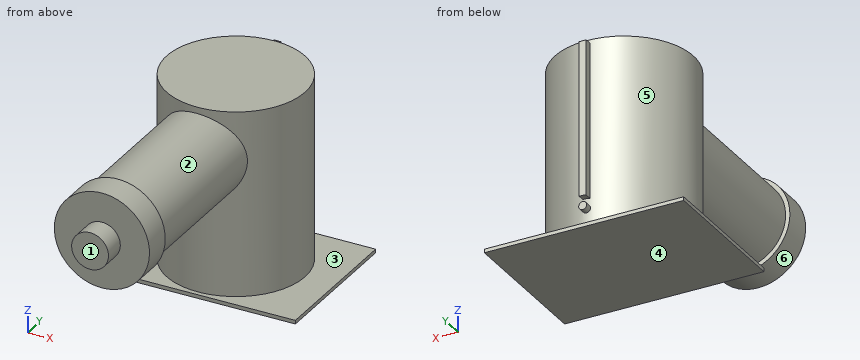
from build123d import *

# Parameters (mm, degrees)
SKETCH2_W           = 54.93072207
SKETCH2_H           = 40.655962058
BOSS_EXTRUDE1_DEPTH = 1
SKETCH3_R           = 19.076133807
BOSS_EXTRUDE2_DEPTH = 51
SKETCH4_R           = 11.934045709
BOSS_EXTRUDE3_DEPTH = 40
BOSS_EXTRUDE4_START = 10
SKETCH5_R           = 11.934045709
BOSS_EXTRUDE4_DEPTH = 10
SKETCH6_R           = 13.112340193
BOSS_EXTRUDE5_DEPTH = 8
SKETCH7_R           = 5.071080503
BOSS_EXTRUDE6_DEPTH = 6
SKETCH8_R           = 1.107443945
BOSS_EXTRUDE7_DEPTH = 2
SCALE1_SCALE        = 0.5
SCALE2_SCALE        = 0.5
SCALE3_SCALE        = 0.5


with BuildPart() as part:
    # Sketch2 → Boss-Extrude1 (new body)
    with BuildSketch(Plane.XY):
        Rectangle(SKETCH2_W, SKETCH2_H)
    extrude(amount=BOSS_EXTRUDE1_DEPTH)

    # Sketch3 → Boss-Extrude2 (add)
    with BuildSketch(Plane.XY.offset(1)):
        Circle(SKETCH3_R)
    extrude(amount=BOSS_EXTRUDE2_DEPTH)

    # Sketch4 → Boss-Extrude3 (add)
    with BuildSketch(Plane(origin=(0, -19, 0), x_dir=(1, 0, 0), z_dir=(0, 1, 0))):
        with Locations(Location((-0.455521122, -38.326598174, 0), (0, 0, 270))):
            Circle(SKETCH4_R)
    extrude(amount=-BOSS_EXTRUDE3_DEPTH)

    # Sketch5 → Boss-Extrude4 (add)
    with BuildSketch(Plane(origin=(0, -19, 0), x_dir=(1, 0, 0), z_dir=(0, 1, 0)).offset(BOSS_EXTRUDE4_START)):
        with Locations(Location((-0.455521122, -38.326598174, 0), (0, 0, 270))):
            Circle(SKETCH5_R)
    extrude(amount=-BOSS_EXTRUDE4_DEPTH)

    # Sketch6 → Boss-Extrude5 (add)
    with BuildSketch(Plane.XZ.offset(59)):
        with Locations(Location((-0.455521122, 38.326598174, 0), (0, 0, 270))):
            Circle(SKETCH6_R)
    extrude(amount=BOSS_EXTRUDE5_DEPTH)

    # Sketch7 → Boss-Extrude6 (add)
    with BuildSketch(Plane.XZ.offset(67)):
        with Locations(Location((-0.455521122, 38.326598174, 0), (0, 0, 270))):
            Circle(SKETCH7_R)
    extrude(amount=BOSS_EXTRUDE6_DEPTH)

    # Sketch8 → Boss-Extrude7 (add)
    with BuildSketch(Plane(origin=(0, 19, 0), x_dir=(1, 0, 0), z_dir=(0, 1, 0))):
        with BuildLine():
            add(Edge.make_bspline(
                [(-0.976975476, -8.151409565), (-0.015117663, -8.40988659), (0.976975476, -8.324614056)],
                knots=[0, 0, 0, 1, 1, 1], degree=2))
            Line((0.976975476, -8.324614056), (0.976975476, -51.031726638))
            Line((0.976975476, -51.031726638), (-0.976975476, -51.031726638))
            Line((-0.976975476, -51.031726638), (-0.976975476, -8.151409565))
        make_face()
        with Locations(Location((0, -5.474365912, 0), (0, 0, 90))):
            Circle(SKETCH8_R)
    extrude(amount=BOSS_EXTRUDE7_DEPTH)


with BuildPart() as part_1:
    # Scale1: scaled about (0, 0, 0)
    add(part.part.scale(SCALE1_SCALE))


with BuildPart() as part_2:
    # Scale2: scaled about (0, 0, 0)
    add(part_1.part.scale(SCALE2_SCALE))


with BuildPart() as part_3:
    # Scale3: scaled about (0, 0, 0)
    add(part_2.part.scale(SCALE3_SCALE))


solid = part_3.part
Geometry: final body of the model. Coordinates: model frame, mm. Face numbers are marked on the shaded views. A direction names the side the tool comes from. Coordinates: 2 decimals unless noted, no trailing zeros. Order: outer loops, then holes, each group sorted by start corner. A loop starts at its lowest first (then second) coordinate and runs counter-clockwise, first axis right, second up.
1) Set-up query: the marked faces 4, 5 and 6. Return all of +Z, -Z, +X, -X, +Y, -Y with unobstructed straight access to the full face (end or side cutting, diameter ignored); none if empty.
Result sheet:
face 4: -Z, +X, -X, +Y, -Y
face 5: none
face 6: -Y
2) Ray query, probe 1 along Y at (x, z) = (0, 2.75) (3 decimals); probe 2 along Y at (x, z) = (-1, 3.5) (3 decimals); probe 3 along Z at (x, y) = (-0.25, -5.5). Return the intervals inside material, ascending.
Result sheet:
probe 1: y = -2.385 to 2.625
probe 2: y = -8.375 to -7.375, -2.165 to 2.165
probe 3: z = 3.31 to 6.27
3) Section A-A (y = 0). Return loops of the section in (x, z) (3 decimals).
Result sheet:
outline: (-3.433, 0) - (3.433, 0) - (3.433, 0.125) - (2.385, 0.125) - (2.385, 6.5) - (-2.385, 6.5) - (-2.385, 0.125) - (-3.433, 0.125) - close
4) Section C-C (x = -2.25). Return loops of the section in (y, z) (3 decimals).
Result sheet:
outline: (-2.541, 0) - (2.541, 0) - (2.541, 0.125) - (0.79, 0.125) - (0.79, 6.5) - (-0.79, 6.5) - (-0.79, 0.125) - (-2.541, 0.125) - close
5) First-contact query: P1, Ø3, axis at x = 1.5, z = 1, coming from the -Y side; P2, Ø1, axis at x = 1.5, z = 5.5, coming from the +Y side; P3, Ø3, axis at x = -0.5, y = -4, coming from the +Z side. Flat tips, straight axial feed; report the tip coordinate or a pass-through.
Result sheet:
P1: stops at y = -2.54
P2: stops at y = 2.16
P3: stops at z = 6.28
6) Section D-D (x = -1). Return loops of the section in (y, z) (3 decimals), then the cut area to 3 significant figures.
Result sheet:
outline: (-8.375, 3.45) - (-7.375, 3.45) - (-7.375, 3.635) - (-2.165, 3.635) - (-2.165, 0.125) - (-2.541, 0.125) - (-2.541, 0) - (2.541, 0) - (2.541, 0.125) - (2.165, 0.125) - (2.165, 6.5) - (-2.165, 6.5) - (-2.165, 5.947) - (-7.375, 5.947) - (-7.375, 6.131) - (-8.375, 6.131) - close
area: 43.0 mm2
7) Draft query along Y for the marked faces 1, 2 and 3. Return one class per face: released by +Y, released by -Y, zero draft, split by the parting line, or undercut.
Result sheet:
face 1: released by -Y
face 2: undercut
face 3: zero draft
